```python
from build123d import *

# Parameters (mm, degrees)
CROQUIS1_W              = 500
CROQUIS1_H              = 58
SALIENTE_EXTRUIR1_DEPTH = 2
CROQUIS4_W              = 500
CROQUIS4_H              = 2
SALIENTE_EXTRUIR2_DEPTH = 3
REDONDEO1_R             = 2


with BuildPart() as part:
    # Croquis1 → Saliente-Extruir1 (new body)
    with BuildSketch(Plane(origin=(0, 0, 0), x_dir=(1, 0, 0), z_dir=(0, 1, 0))):
        Rectangle(CROQUIS1_W, CROQUIS1_H)
    extrude(amount=SALIENTE_EXTRUIR1_DEPTH)

    # Croquis4 → Saliente-Extruir2 (add)
    with BuildSketch(Plane(origin=(0, 0, 0), x_dir=(1, 0, 0), z_dir=(0, 1, 0))):
        with Locations((0, 30)):
            Rectangle(CROQUIS4_W, CROQUIS4_H)
        with Locations((0, -30)):
            Rectangle(CROQUIS4_W, CROQUIS4_H)
    extrude(amount=SALIENTE_EXTRUIR2_DEPTH)

    # Redondeo1
    # the kernel refuses this fillet: 2 mm, written as the material it takes off along each edge
    with BuildSketch(Plane(origin=(254.330127019, 3, -29), x_dir=(0, 0, -1), z_dir=(-1, 0, 0))) as redondeo1_piece_1:
        with BuildLine():
            CenterArc((1.732050808, 2), REDONDEO1_R, 210, 60)
            Line((0, 1), (-0.034641016, 0.98))
            ThreePointArc((-0.034641016, 0.98), (-0.04, 0.5), (-0.04, 0))
            Line((-0.04, 0), (0, -0.04))
            Line((0, -0.04), (1.732050808, -0.04))
            Line((1.732050808, -0.04), (1.732050808, 0))
        make_face()
    extrude(amount=508.660254038, mode=Mode.SUBTRACT)
    with BuildSketch(Plane(origin=(-254.330127019, 3, 29), x_dir=(0, -1, 0), z_dir=(1, 0, 0))) as redondeo1_piece_2:
        with BuildLine():
            CenterArc((2, -1.732050808), REDONDEO1_R, 120, 60)
            Line((0, -1.732050808), (-0.04, -1.732050808))
            Line((-0.04, -1.732050808), (-0.04, 0))
            Line((-0.04, 0), (0, 0.04))
            ThreePointArc((0, 0.04), (0.5, 0.04), (0.98, 0.034641016))
            Line((0.98, 0.034641016), (1, 0))
        make_face()
    extrude(amount=508.660254038, mode=Mode.SUBTRACT)


solid = part.part
```
The listing builds one solid part. Answer for the finished solid, in the listing's coordinates (mm). Coordinates: 2 decimals unless noted, no trailing zeros. Loops run counter-clockwise (first coordinate to the right, second up) from the corner with the lowest first, then second, coordinate; pieces in that order, holes last. Notation, with made-up numbers: M -21.5,-33.75 L -1.5,-33.75 A20 cw -1.5,-5.75 Z; hole C -33,15.5 d10. An arc over 180 degrees is marked long. Answer as CSV lines item,"result". Start each with the question number.
(1) The part is cut by section B-B (y = 2.55). Give the vertices of the cut face in (x, z).
(2) The part is cut by section A-A (x = 217). Give the vertices of the cut face in (y, z), and give its area (3 significant figures).
(3) The mould has two halves that part along Z. Classify faces 1 (the flat face through (-3, 2, 0)), 2 (the flat face through (-3, 0, 0)): pulls with the +Z half, pulls with the -Z half, needs draft (parallel to the pull), parting line crosses it, or undercut.
(4) Find the intervals of material crossed by L1, parallel to Z at x = 186.5, y = 2.15; L2, parallel to Y at x = -16.5, z = 7.5, in increasing order. Write a range as [from, to].
(5) Given pin 1 (3 mm diameter, centred on x = -138, z = -15, fed in from +Y), flat-ended and moving along its own axis, determine where the tip first touches the part or whether it passes through.
(6) The part is cut by section C-C (z = 13). Give the vertices of the cut face in (x, y), and give its area (3 significant figures).
Determined:
1,outline,"M -250,-31 L 250,-31 L 250,-29.47 L -250,-29.47 Z; M -250,29.47 L 250,29.47 L 250,31 L -250,31 Z"
2,outline,"M 0,-31 L 3,-31 L 3,-30.73 A2 ccw 2,-29 L 2,29 A2 ccw 3,30.73 L 3,31 L 0,31 Z"
2,area,"127 mm2"
3,face 1,"undercut"
3,face 2,"needs draft"
4,L1,"[-31, -29.1], [29.1, 31]"
4,L2,"[0, 2]"
5,pin 1,"y = 2"
6,outline,"M -250,0 L 250,0 L 250,2 L -250,2 Z"
6,area,"1,000 mm2"
